Input: dimensioned drawing with shaded views. Units: mm. Origin: part minimum x, y, z. A direction names the side the tool comes from. Give positions to 0.01 mm unless a question says otherwise; leave off trailing zeros. Write each loop counter-clockwise with the first axis right and the second up, starting at its lowest first coordinate (ties: lowest second). Pieces come first, ordered by that corner, then holes.
Q1. Section B-B (x = 22.5). Return the cut outline in (y, z), plus the area to 3 significant figures.
Q2. Section D-D (x = 10). Return the cut outline in (y, z).
Q3. Line query: line 1 (Z direction, x = 39.3, y = 1.4); line 2 (X direction, y = 1.55, z = 12); line 3 (Y direction, x = 10, z = 9.25). Output: solid intervals per line, ascending.
Q4. Reachability of the marked faces 1 and 2 from +Z, -Z, +X, -X, +Y, -Y: full face, straight path, thin tool, end or side. Return the list, or none.
Q5. Section A-A (y = 13.15). Return the cut outline in (x, z) (3 decimals).
Q6. Section C-C (z = 12). Return the cut outline in (x, y), plus the area to 4 significant figures.
Q7. Pin query (flat end, axial travel): pin 1 Ø3 at (x, z) = (39.3, 12) entering from +Y; pin 2 Ø8 at (x, z) = (20.5, 10) entering from +Y; pin 3 Ø4 at (x, y) = (12, 7.5) entering from +Z; pin 4 Ø6.5 at (x, y) = (27, 14) entering from +Z. Return the tip coordinate at first contact, or that it passes through.
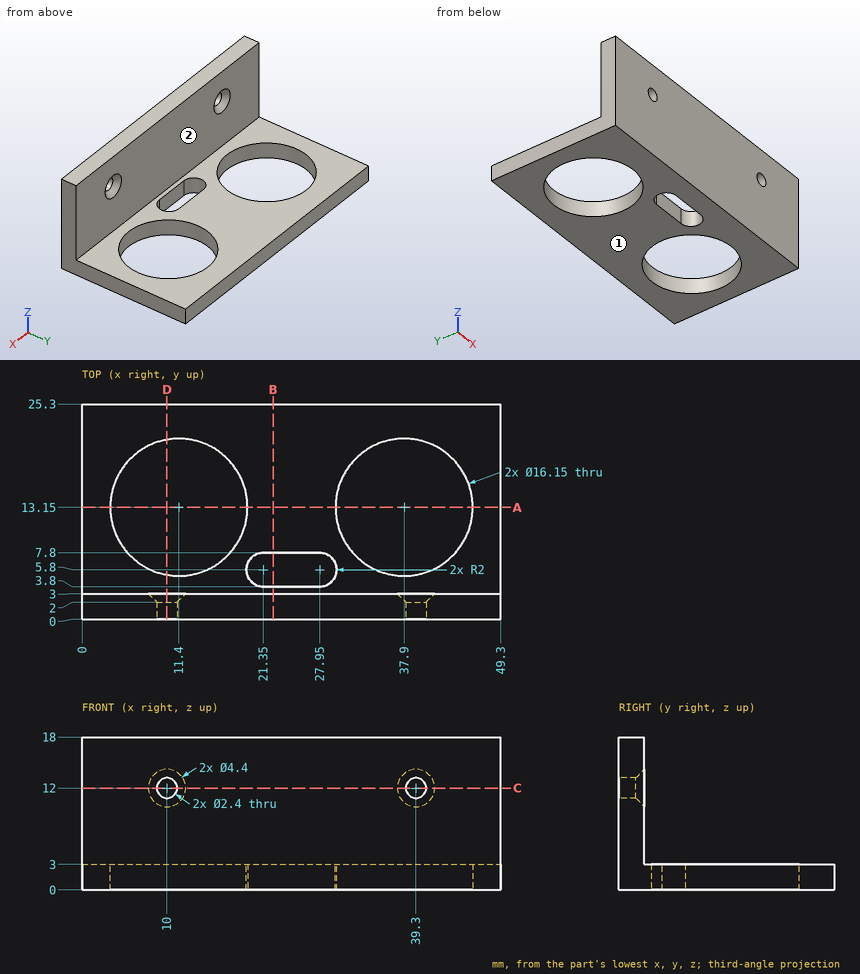
Computed:
1. outline: (0, 0) - (3.8, 0) - (3.8, 3) - (3, 3) - (3, 18) - (0, 18) - close; (7.8, 0) - (25.3, 0) - (25.3, 3) - (7.8, 3) - close
1. area: 109 mm2
2. outline: (0, 0) - (5.2, 0) - (5.2, 3) - (3, 3) - (3, 9.8) - (2, 10.8) - (0, 10.8) - close; (0, 13.2) - (2, 13.2) - (3, 14.2) - (3, 18) - (0, 18) - close; (21.1, 0) - (25.3, 0) - (25.3, 3) - (21.1, 3) - close
3. line 1: z = 0 to 10.8, 13.2 to 18
3. line 2: x = 0 to 8.8, 11.2 to 38.1, 40.5 to 49.3
3. line 3: y = 0 to 3
4. face 1: -Z, +X, -X, +Y, -Y
4. face 2: +Z, +X, -X, +Y
5. outline: (0, 0) - (3.325, 0) - (3.325, 3) - (0, 3) - close; (19.475, 0) - (29.825, 0) - (29.825, 3) - (19.475, 3) - close; (45.975, 0) - (49.3, 0) - (49.3, 3) - (45.975, 3) - close
6. outline: (0, 0) - (8.8, 0) - (8.8, 2) - (7.8, 3) - (0, 3) - close; (11.2, 0) - (38.1, 0) - (38.1, 2) - (37.1, 3) - (12.2, 3) - (11.2, 2) - close; (40.5, 0) - (49.3, 0) - (49.3, 3) - (41.5, 3) - (40.5, 2) - close
6. area: 131.5 mm2
7. pin 1: stops at y = 2.3
7. pin 2: stops at y = 3
7. pin 3: passes through
7. pin 4: stops at z = 3
